```python
from build123d import *

# Parameters (mm, degrees)
SKETCH1_W           = 300
SKETCH1_H           = 240
SKETCH1_R           = 1.5
SKETCH1_R_2         = 1.6
SKETCH1_W_2         = 31.4
SKETCH1_H_2         = 15.09
BOSS_EXTRUDE1_DEPTH = 5
SKETCH3_R           = 1.5
CUT_EXTRUDE1_DEPTH  = 385.219989069
SKETCH5_R           = 4
CUT_EXTRUDE3_DEPTH  = 385.219989069
SKETCH8_R           = 4
CUT_EXTRUDE4_DEPTH  = 385.219989069


with BuildPart() as part:
    # Sketch1 → Boss-Extrude1 (new body)
    with BuildSketch(Plane.XY):
        with Locations((150, 120)):
            Rectangle(SKETCH1_W, SKETCH1_H)
        with Locations((7.5, 232.5)):
            Circle(SKETCH1_R, mode=Mode.SUBTRACT)
        with Locations(Location((292.5, 232.5, 0), (0, 0, 180))):
            Circle(SKETCH1_R, mode=Mode.SUBTRACT)
        with Locations((292.5, 7.5)):
            Circle(SKETCH1_R, mode=Mode.SUBTRACT)
        with Locations(Location((7.5, 7.5, 0), (0, 0, 180))):
            Circle(SKETCH1_R, mode=Mode.SUBTRACT)
        with Locations(Location((137, 156.83, 0), (0, 0, 180))):
            Circle(SKETCH1_R_2, mode=Mode.SUBTRACT)
        with Locations((43, 156.83)):
            Circle(SKETCH1_R_2, mode=Mode.SUBTRACT)
        with Locations(Location((43, 83.17, 0), (0, 0, 180))):
            Circle(SKETCH1_R_2, mode=Mode.SUBTRACT)
        with Locations((137, 83.17)):
            Circle(SKETCH1_R_2, mode=Mode.SUBTRACT)
        with Locations((90, 181.375)):
            Rectangle(SKETCH1_W_2, SKETCH1_H_2, mode=Mode.SUBTRACT)
        with Locations((90, 58.625)):
            Rectangle(SKETCH1_W_2, SKETCH1_H_2, mode=Mode.SUBTRACT)
    extrude(amount=BOSS_EXTRUDE1_DEPTH)

    # Sketch3 → Cut-Extrude1 (cut, through all)
    with BuildSketch(Plane.XY.offset(5)):
        with Locations(Location((17.484796486, 136, 0), (0, 0, 180))):
            Circle(SKETCH3_R)
        with Locations(Location((17.484796486, 120, 0), (0, 0, 180))):
            Circle(SKETCH3_R)
        with Locations(Location((17.484796486, 104, 0), (0, 0, 180))):
            Circle(SKETCH3_R)
    extrude(amount=-CUT_EXTRUDE1_DEPTH, mode=Mode.SUBTRACT)

    # Sketch5 → Cut-Extrude3 (cut, through all)
    with BuildSketch(Plane.XY.offset(5)):
        with Locations((194.442432224, 178.625000137)):
            Circle(SKETCH5_R)
        with Locations((228.442432224, 178.625000137)):
            Circle(SKETCH5_R)
        with Locations((262.442432224, 178.625000137)):
            Circle(SKETCH5_R)
    extrude(amount=-CUT_EXTRUDE3_DEPTH, mode=Mode.SUBTRACT)

    # Sketch8 → Cut-Extrude4 (cut, through all)
    with BuildSketch(Plane.XY.offset(5)):
        with Locations((194.442432224, 61.375000137)):
            Circle(SKETCH8_R)
        with Locations((228.442432224, 61.375000137)):
            Circle(SKETCH8_R)
        with Locations((262.442432224, 61.375000137)):
            Circle(SKETCH8_R)
    extrude(amount=-CUT_EXTRUDE4_DEPTH, mode=Mode.SUBTRACT)


solid = part.part
```
Check sheet for the modelled part. Datum: model origin and axes. Units: mm. Coordinates: 2 decimals unless noted, no trailing zeros. Write item = value, one per line. Start each with the question number.
1) Mould release check, pull along Y, two halves, no side actions. Record for faces 1 (the flat face through (148, 122, 5)), 2 (the cylindrical face through (264.59, 64.75, 2.54)): +Y half, -Y half, draft (parallel to the pull), parting line (faces both ways), or undercut.
2) Cross-section at A-A (z = 2). State how many separate pieces and enclosed holes the cut face has, then the cut area to 3 significant figures.
3) Material ranges on L1, parallel to Y at x = 292.5, z = 1.3; L2, parallel to X at y = 156.83, z = 3.7; L3, parallel to Y at x = 105, z = 1.5, recorded low to high.
Ans:
q1.face_1 = draft
q1.face_2 = undercut
q2.separate_pieces = 1
q2.enclosed_holes = 19
q2.area = 70,700 mm²
q3.L1 = 0 to 6, 9 to 231, 234 to 240
q3.L2 = 0 to 41.4, 44.6 to 135.4, 138.6 to 300
q3.L3 = 0 to 51.08, 66.17 to 173.83, 188.92 to 240
